Could you check a few things on this model? Use its own coordinates, in mm. Coordinates: 2 decimals unless noted, no trailing zeros. Loops run counter-clockwise (first coordinate to the right, second up) from the corner with the lowest first, then second, coordinate; pieces in that order, holes last. Notation, with made-up numbers: (-17, 45.5) - (8, 45.5) arc R34 cw to (8, 78.5) - close; hole circle Ø3 at (-2, 81.5). An arc over 180 degrees is marked (long way). One line per question, with ' | ' between items. Start each with the question number.
1. I want a section at B-B, the plane y = 671.5. Write out the boundary of the cut face in (x, z), then the cut area to 3 significant figures.
2. I'm going to push flat-ended pins straight in: P1, Ø5, axis at x = 12.7, y = 241.3, coming from the +Z side; P2, Ø6, axis at x = 158.5, z = 1.5, coming from the +Y side; P3, Ø6.5, axis at x = 33, z = 6.5, coming from the -Y side; P4, Ø6, axis at y = 94, z = 2.5, coming from the +X side. Where does each tip first touch, or does it pass through?
3. Please list where these lines run through material, in increasing order: L1, parallel to X at y = 190.5, z = 9.5; L2, parallel to Y at x = 215.9, z = 3; L3, parallel to Y at x = 52, z = 1.25. Write a range as [from, to].
4. I want a section at A-A, the plane z = 5.5. Count the separate pieces of the cut face and the enclosed holes in it, then the cut area to 3 significant figures.
5. I want a section at C-C, the plane x = 125.5. Write out the boundary of the cut face in (y, z).
Autodesk Inventor part; units mm, degrees
ref_plane "YZ Plane" through (0, 0, 0) normal (1, 0, 0) x (0, 1, 0)
ref_plane "XZ Plane" through (0, 0, 0) normal (0, 1, 0) x (-1, 0, 0)
ref_plane "XY Plane" through (0, 0, 0) normal (0, 0, 1) x (1, 0, 0)
ref_plane "Work Plane1" through (0, 0, 0) normal (0, 0, 1) x (1, 0, 0)
sketch "Sketch1" plane through (0, 0, 0) normal (0, 0, 1) x (1, 0, 0)
  circle A0 centre (495.3, 317.5) radius 1.5875
  circle A1 centre (495.3, 698.5) radius 1.5875
  circle A2 centre (495.3, 673.1) radius 1.5875
  circle A3 centre (495.3, 647.7) radius 1.5875
  circle A4 centre (495.3, 622.3) radius 1.5875
  circle A5 centre (495.3, 596.9) radius 1.5875
  circle A6 centre (495.3, 571.5) radius 1.5875
  circle A7 centre (495.3, 546.1) radius 1.5875
  circle A8 centre (495.3, 520.7) radius 1.5875
  circle A9 centre (495.3, 495.3) radius 1.5875
  circle A10 centre (495.3, 469.9) radius 1.5875
  circle A11 centre (495.3, 444.5) radius 1.5875
  circle A12 centre (495.3, 419.1) radius 1.5875
  circle A13 centre (495.3, 393.7) radius 1.5875
  circle A14 centre (495.3, 368.3) radius 1.5875
  circle A15 centre (495.3, 342.9) radius 1.5875
  circle A16 centre (495.3, 317.5) radius 1.5875
  circle A17 centre (495.3, 292.1) radius 1.5875
  circle A18 centre (495.3, 266.7) radius 1.5875
  circle A19 centre (495.3, 241.3) radius 1.5875
  circle A20 centre (495.3, 215.9) radius 1.5875
  circle A21 centre (495.3, 190.5) radius 1.5875
  circle A22 centre (495.3, 165.1) radius 1.5875
  circle A23 centre (495.3, 139.7) radius 1.5875
  circle A24 centre (495.3, 114.3) radius 1.5875
  circle A25 centre (495.3, 88.9) radius 1.5875
  circle A26 centre (495.3, 63.5) radius 1.5875
  circle A27 centre (495.3, 38.1) radius 1.5875
  circle A28 centre (495.3, 12.7) radius 1.5875
  line L0 (482.6, 0) -> (508, 0)
  line L1 (508, 0) -> (508, 711.2)
  line L2 (482.6, 711.2) -> (508, 711.2)
  line L3 (482.6, 0) -> (482.6, 711.2)
  circle A29 centre (469.9, 723.9) radius 1.5875
  circle A30 centre (444.5, 723.9) radius 1.5875
  circle A31 centre (419.1, 723.9) radius 1.5875
  circle A32 centre (393.7, 723.9) radius 1.5875
  circle A33 centre (368.3, 723.9) radius 1.5875
  circle A34 centre (342.9, 723.9) radius 1.5875
  circle A35 centre (317.5, 723.9) radius 1.5875
  circle A36 centre (292.1, 723.9) radius 1.5875
  circle A37 centre (266.7, 723.9) radius 1.5875
  circle A38 centre (241.3, 723.9) radius 1.5875
  circle A39 centre (215.9, 723.9) radius 1.5875
  circle A40 centre (190.5, 723.9) radius 1.5875
  circle A41 centre (165.1, 723.9) radius 1.5875
  circle A42 centre (139.7, 723.9) radius 1.5875
  circle A43 centre (114.3, 723.9) radius 1.5875
  circle A44 centre (88.9, 723.9) radius 1.5875
  circle A45 centre (63.5, 723.9) radius 1.5875
  circle A46 centre (38.1, 723.9) radius 1.5875
  line L4 (25.4, 736.6) -> (25.4, 711.2)
  line L5 (25.4, 711.2) -> (482.6, 711.2)
  line L6 (482.6, 736.6) -> (482.6, 711.2)
  line L7 (25.4, 736.6) -> (482.6, 736.6)
  circle A47 centre (38.1, -12.7) radius 1.5875
  circle A48 centre (63.5, -12.7) radius 1.5875
  circle A49 centre (88.9, -12.7) radius 1.5875
  circle A50 centre (114.3, -12.7) radius 1.5875
  circle A51 centre (139.7, -12.7) radius 1.5875
  circle A52 centre (165.1, -12.7) radius 1.5875
  circle A53 centre (190.5, -12.7) radius 1.5875
  circle A54 centre (215.9, -12.7) radius 1.5875
  circle A55 centre (241.3, -12.7) radius 1.5875
  circle A56 centre (266.7, -12.7) radius 1.5875
  circle A57 centre (292.1, -12.7) radius 1.5875
  circle A58 centre (317.5, -12.7) radius 1.5875
  circle A59 centre (342.9, -12.7) radius 1.5875
  circle A60 centre (368.3, -12.7) radius 1.5875
  circle A61 centre (393.7, -12.7) radius 1.5875
  circle A62 centre (419.1, -12.7) radius 1.5875
  circle A63 centre (444.5, -12.7) radius 1.5875
  circle A64 centre (469.9, -12.7) radius 1.5875
  line L8 (482.6, -25.4) -> (482.6, 0)
  line L9 (482.6, 0) -> (25.4, 0)
  line L10 (25.4, -25.4) -> (25.4, 0)
  line L11 (482.6, -25.4) -> (25.4, -25.4)
  circle A65 centre (12.7, 698.5) radius 1.5875
  circle A66 centre (12.7, 673.1) radius 1.5875
  circle A67 centre (12.7, 647.7) radius 1.5875
  circle A68 centre (12.7, 622.3) radius 1.5875
  circle A69 centre (12.7, 596.9) radius 1.5875
  circle A70 centre (12.7, 571.5) radius 1.5875
  circle A71 centre (12.7, 546.1) radius 1.5875
  circle A72 centre (12.7, 520.7) radius 1.5875
  circle A73 centre (12.7, 495.3) radius 1.5875
  circle A74 centre (12.7, 469.9) radius 1.5875
  circle A75 centre (12.7, 444.5) radius 1.5875
  circle A76 centre (12.7, 419.1) radius 1.5875
  circle A77 centre (12.7, 393.7) radius 1.5875
  circle A78 centre (12.7, 368.3) radius 1.5875
  circle A79 centre (12.7, 342.9) radius 1.5875
  circle A80 centre (12.7, 317.5) radius 1.5875
  circle A81 centre (12.7, 292.1) radius 1.5875
  circle A82 centre (12.7, 266.7) radius 1.5875
  circle A83 centre (12.7, 241.3) radius 1.5875
  circle A84 centre (12.7, 215.9) radius 1.5875
  circle A85 centre (12.7, 190.5) radius 1.5875
  circle A86 centre (12.7, 165.1) radius 1.5875
  circle A87 centre (12.7, 139.7) radius 1.5875
  circle A88 centre (12.7, 114.3) radius 1.5875
  circle A89 centre (12.7, 88.9) radius 1.5875
  circle A90 centre (12.7, 63.5) radius 1.5875
  circle A91 centre (12.7, 38.1) radius 1.5875
  circle A92 centre (12.7, 12.7) radius 1.5875
  line L12 (0, 0) -> (25.4, 0)
  line L13 (25.4, 0) -> (25.4, 711.2)
  line L14 (0, 711.2) -> (25.4, 711.2)
  line L15 (0, 0) -> (0, 711.2)
  line L16 (0, 533.4) -> (0, 177.8)
  line L17 (508, 177.8) -> (508, 533.4)
  line L18 (304.8, 736.6) -> (203.2, 736.6)
  line L19 (203.2, -25.4) -> (304.8, -25.4)
  line L20 (428.9731, 177.8) -> (304.8, 53.6269)
  spline S0 degree 3 number of poles 75
  line L21 (429.7528, 155.0822) -> (327.5178, 52.8472)
  line L22 (82.5441, 177.8) -> (203.2, 57.1441)
  line L23 (180.4822, 52.8472) -> (78.2472, 155.0822)
  line L24 (203.2, 656.5375) -> (80.0625, 533.4)
  line L25 (78.2472, 556.1178) -> (180.4822, 658.3528)
  line L26 (327.5178, 658.3528) -> (429.7528, 556.1178)
  line L27 (304.8, 658.3528) -> (429.7528, 533.4)
  line L28 (203.2, 736.6) -> (203.2, 656.5375)
  line L29 (203.2, 57.1441) -> (203.2, -25.4)
  line L30 (304.8, 658.3528) -> (304.8, 736.6)
  line L31 (508, 533.4) -> (429.7528, 533.4)
  line L32 (80.0625, 533.4) -> (0, 533.4)
  line L33 (0, 177.8) -> (82.5441, 177.8)
  line L34 (428.9731, 177.8) -> (508, 177.8)
  line L35 (304.8, -25.4) -> (304.8, 53.6269)
extrude "Extrusion1" add sketch "Sketch1" along normal blind 12.7 contours A0 | A8 | A9 | A10 | A11 | A12 | A13 | A14 | A15 | A17 | A18 | A19 | A20 | A21 | L34 L20 L35 L9 L29 L22 L33 L13 L32 L24 L28 L5 L30 L27 L31 L3 | L3 L31 L1 L34 | L35 L11 L29 L9 | L5 L28 L7 L30 | L33 L15 L32 L13 | A36 | A37 | A38 | A39 | A54 | A55 | A56 | A57 | A72 | A73 | A74 | A75 | A76 | A77 | A78 | A79 | A80 | A81 | A82 | A83 | A84 | A85
sketch "Sketch2" plane through (0, 0, 0) normal (0, 0, -1) x (-1, 0, 0)
  circle A0 centre (-495.3, 190.5) radius 1.5875
  circle A1 centre (-495.3, 215.9) radius 1.5875
  circle A2 centre (-495.3, 241.3) radius 1.5875
  circle A3 centre (-495.3, 266.7) radius 1.5875
  circle A4 centre (-495.3, 292.1) radius 1.5875
  circle A5 centre (-495.3, 317.5) radius 1.5875
  circle A6 centre (-495.3, 342.9) radius 1.5875
  circle A7 centre (-495.3, 368.3) radius 1.5875
  circle A8 centre (-495.3, 393.7) radius 1.5875
  circle A9 centre (-495.3, 419.1) radius 1.5875
  circle A10 centre (-495.3, 444.5) radius 1.5875
  circle A11 centre (-495.3, 469.9) radius 1.5875
  circle A12 centre (-495.3, 495.3) radius 1.5875
  circle A13 centre (-495.3, 520.7) radius 1.5875
  circle A14 centre (-215.9, 723.9) radius 1.5875
  circle A15 centre (-241.3, 723.9) radius 1.5875
  circle A16 centre (-266.7, 723.9) radius 1.5875
  circle A17 centre (-292.1, 723.9) radius 1.5875
  circle A18 centre (-12.7, 520.7) radius 1.5875
  circle A19 centre (-12.7, 495.3) radius 1.5875
  circle A20 centre (-12.7, 469.9) radius 1.5875
  circle A21 centre (-12.7, 444.5) radius 1.5875
  circle A22 centre (-12.7, 419.1) radius 1.5875
  circle A23 centre (-12.7, 393.7) radius 1.5875
  circle A24 centre (-12.7, 368.3) radius 1.5875
  circle A25 centre (-12.7, 342.9) radius 1.5875
  circle A26 centre (-12.7, 317.5) radius 1.5875
  circle A27 centre (-12.7, 292.1) radius 1.5875
  circle A28 centre (-12.7, 266.7) radius 1.5875
  circle A29 centre (-12.7, 241.3) radius 1.5875
  circle A30 centre (-12.7, 215.9) radius 1.5875
  circle A31 centre (-12.7, 190.5) radius 1.5875
  circle A32 centre (-215.9, -12.7) radius 1.5875
  circle A33 centre (-241.3, -12.7) radius 1.5875
  circle A34 centre (-266.7, -12.7) radius 1.5875
  circle A35 centre (-292.1, -12.7) radius 1.5875
  point P0 (0, 0)
extrude "Extrusion2" cut sketch "Sketch2" against normal blind 12.7
properties part number "baseplate"
Results are:
1) outline: (203.2, 0) - (304.8, 0) - (304.8, 12.7) - (203.2, 12.7) - close | area: 1,290 mm2
2) P1: stops at z = 12.7 | P2: stops at y = 614.84 | P3: stops at y = 177.8 | P4: stops at x = 348.17
3) L1: x = [0, 11.11], [14.29, 493.71], [496.89, 508] | L2: y = [-25.4, -14.29], [-11.11, 722.31], [725.49, 736.6] | L3: y = [177.8, 533.4]
4) separate pieces: 1 | enclosed holes: 36 | area: 252,000 mm2
5) outline: (134.84, 0) - (578.84, 0) - (578.84, 12.7) - (134.84, 12.7) - close
